Study the drawing (mm; zero at the part's minimum x, y, z) and answer. A direction names the side the tool comes from. Round coordinates to 2 decimals unless told otherwise and drop trailing zeros. Loops run counter-clockwise (first coordinate to the right, second up) from the corner with the lowest first, then second, coordinate; pieces in that order, holes last. Notation, with made-up numbers: (17, 4.5) - (40, 4.5) arc R24 ccw to (40, 32.5) - close; hole circle Ø1 at (66.5, -31.75). An arc over 180 degrees is marked (long way). One line per item, written item: value.
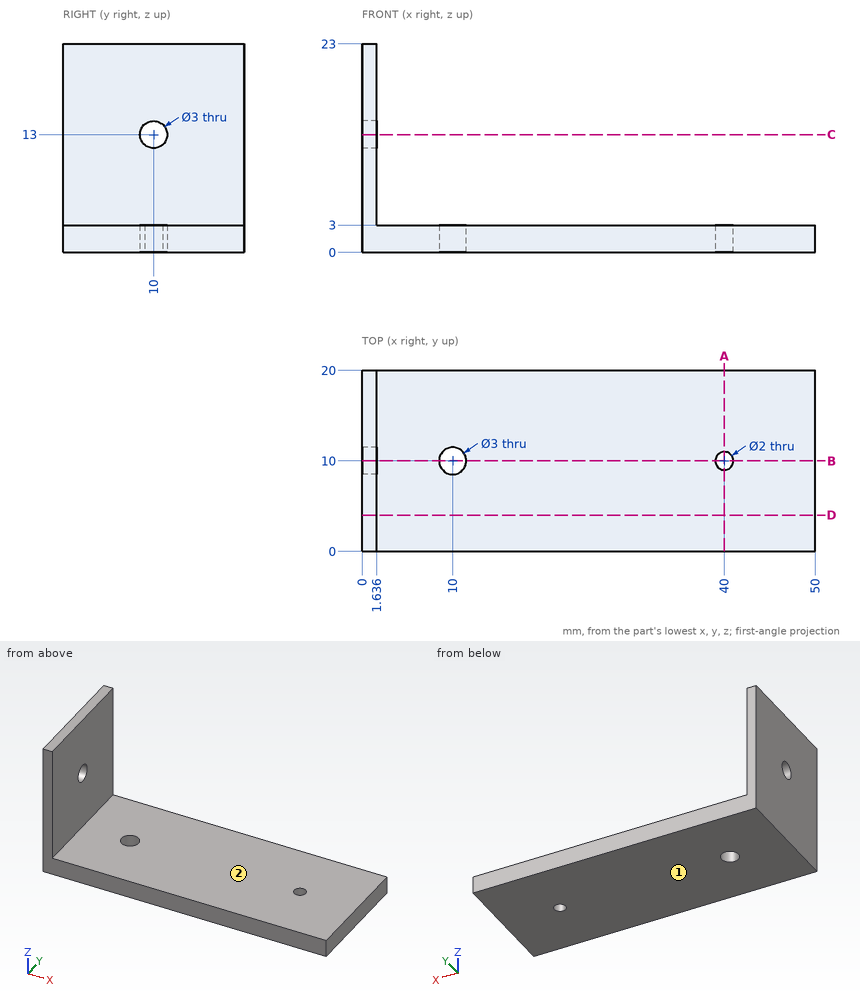
1) For the marked faces 1 and 2, determine the directions among +Z, -Z, +X, -X, +Y, -Y from which every point of the face is accessible in a straight line to the end or side of a thin tool.
Final values:
face 1: -Z, +X, -X, +Y, -Y
face 2: +Z, +X, +Y, -Y
2) A cutting plane is placed at B-B on y = 10. Give the vertices of the cut face in (x, z), and give its area (3 significant figures).
Final values:
outline: (0, 0) - (8.5, 0) - (8.5, 3) - (1.64, 3) - (1.64, 11.5) - (0, 11.5) - close; (0, 14.5) - (1.64, 14.5) - (1.64, 23) - (0, 23) - close; (11.5, 0) - (39, 0) - (39, 3) - (11.5, 3) - close; (41, 0) - (50, 0) - (50, 3) - (41, 3) - close
area: 163 mm2
3) Each of these flat-tipped pins is pushed along its axis until it touches: pin 1 Ø6 at (y, z) = (12, 17.5) entering from +X; pin 2 Ø10 at (x, y) = (15, 7.5) entering from +Z. Where does it stop, or does it pass through?
Final values:
pin 1: x = 1.64
pin 2: z = 3
4) A cutting plane is placed at A-A on x = 40. Give the vertices of the cut face in (y, z), and give its area (3 significant figures).
Final values:
outline: (0, 0) - (9, 0) - (9, 3) - (0, 3) - close; (11, 0) - (20, 0) - (20, 3) - (11, 3) - close
area: 54.0 mm2
5) Consider L1, parallel to X at y = 9.25, z = 1.5; L2, parallel to Y at x = 10, z = 1.4; L3, parallel to X at y = 19.25, z = 5.5. Determine where each line is inside the solid, lowest interval first.
Final values:
L1: 0 to 8.7, 11.3 to 39.34, 40.66 to 50
L2: 0 to 8.5, 11.5 to 20
L3: 0 to 1.64
6) A cutting plane is placed at C-C on z = 13. Give the vertices of the cut face in (x, y).
Final values:
outline: (0, 0) - (1.64, 0) - (1.64, 8.5) - (0, 8.5) - close; (0, 11.5) - (1.64, 11.5) - (1.64, 20) - (0, 20) - close
7) A cutting plane is placed at D-D on y = 4. Give the vertices of the cut face in (x, z), and give its area (3 significant figures).
Final values:
outline: (0, 0) - (50, 0) - (50, 3) - (1.64, 3) - (1.64, 23) - (0, 23) - close
area: 183 mm2
